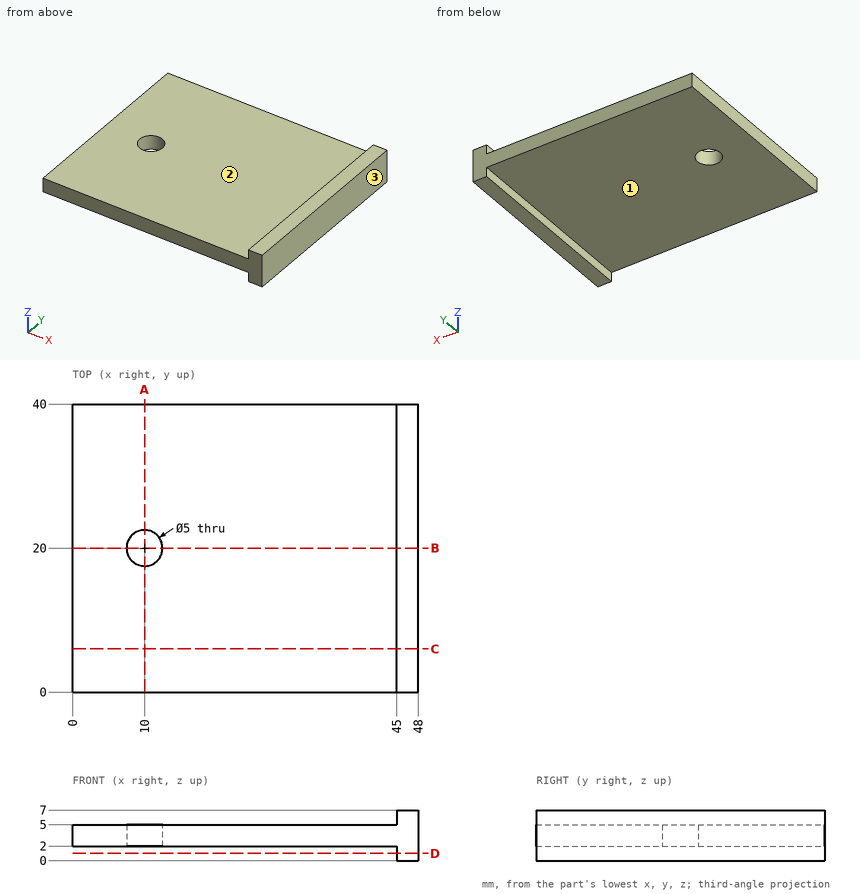
The figure shows three views and two pictorial views of one solid part (mm, origin at its lowest corner). Answer the questions. A direction names the side the tool comes from. Give positions to 0.01 mm unless a question says otherwise; leave off trailing zeros. Order: outer loops, then holes, each group sorted by start corner. A loop starts at its lowest first (then second) coordinate and runs counter-clockwise, first axis right, second up. Notation, with made-up numbers: (86, 87.5) -> (111, 87.5) arc R23 ccw to (111, 101.5) -> close; hole circle Ø1 at (12, -8.75). An arc over 180 degrees is marked (long way). One line per item, written item: value.
1) A tool of negligible diameter and unlimited length cuts with its end or side. For the marked faces 1, 2 and 3, from which of +Z, -Z, +X, -X, +Y, -Y can it reach the whole face along a straight path? Write none if from no direction.
Reported:
face 1: -Z, -X, +Y, -Y
face 2: +Z, -X, +Y, -Y
face 3: +Z, -Z, +X, +Y, -Y
2) Find section B-B, the plane y = 20. Determine the outline of the cut face in (x, z), plus the area to 3 significant figures.
Reported:
outline: (0, 2) -> (7.5, 2) -> (7.5, 5) -> (0, 5) -> close; (12.5, 2) -> (45, 2) -> (45, 0) -> (48, 0) -> (48, 7) -> (45, 7) -> (45, 5) -> (12.5, 5) -> close
area: 141 mm^2
3) Find section A-A, the plane x = 10. Determine the outline of the cut face in (y, z).
Reported:
outline: (0, 2) -> (17.5, 2) -> (17.5, 5) -> (0, 5) -> close; (22.5, 2) -> (40, 2) -> (40, 5) -> (22.5, 5) -> close
4) Find the intervals of material crossed by line 1 (Y direction, x = 10, z = 4.35); line 2 (Z direction, x = 17.5, y = 38); line 3 (X direction, y = 12, z = 0.75), in increasing order.
Reported:
line 1: y = 0 to 17.5, 22.5 to 40
line 2: z = 2 to 5
line 3: x = 45 to 48
5) Flat-ended cylindrical pins translate along their axes: P1, Ø10, axis at x = 27.5, y = 23, coming from the -Z side; P2, Ø12, axis at x = 13.5, y = 14.5, coming from the +Z side; P3, Ø1, axis at y = 10.5, z = 6, coming from the -X side; P4, Ø4, axis at y = 13, z = 4.5, coming from the -X side. Find the tip coordinate at first contact, or state that the pin passes through.
Reported:
P1: stops at z = 2
P2: stops at z = 5
P3: stops at x = 45
P4: stops at x = 0
6) Find section D-D, the plane z = 1. Determine the outline of the cut face in (x, y), plus the area to 3 significant figures.
Reported:
outline: (45, 0) -> (48, 0) -> (48, 40) -> (45, 40) -> close
area: 120 mm^2
7) Find section C-C, the plane y = 6. Determine the outline of the cut face in (x, z).
Reported:
outline: (0, 2) -> (45, 2) -> (45, 0) -> (48, 0) -> (48, 7) -> (45, 7) -> (45, 5) -> (0, 5) -> close
